```python
from build123d import *

# Parameters (mm, degrees)
F0_R     = 22.425
F1_DEPTH = 1.5
F2_R     = 10.5
F3_DEPTH = 0.25
F4_R     = 4
F5_DEPTH = 48.25
F7_D     = 4
F9_D     = 4
F11_D    = 3.5
F13_D    = 4


with BuildPart() as f1:
    # F0 (on Front) → F1 (new body)
    with BuildSketch(Plane.XZ):
        Circle(F0_R)
    extrude(amount=F1_DEPTH)

    # F2 (on face) → F3 (join)
    with BuildSketch(Plane.XZ.offset(1.5)):
        Circle(F2_R)
    extrude(amount=F3_DEPTH)

    # F4 (on face) → F5 (join)
    with BuildSketch(Plane.XZ.offset(1.75)):
        Circle(F4_R)
    extrude(amount=F5_DEPTH)

    # F7 (through all)
    with Locations(Plane(origin=(0, 0, 0), x_dir=(0, 1, 0), z_dir=(-1, 0, 0))):
        with Locations((-33, 0)):
            Hole(F7_D / 2)

    # F9 (through all)
    with Locations(Plane.YZ):
        with Locations((-33, 0)):
            Hole(F9_D / 2)

    # F11 (through all)
    with Locations(Plane(origin=(0, 0, 0), x_dir=(-1, 0, 0), z_dir=(0, 1, 0))):
        with Locations((0, 14.25), (-12.340862, -7.125), (12.340862, -7.125)):
            Hole(F11_D / 2)

    # F13 (through all)
    with Locations(Plane(origin=(0, 0, 0), x_dir=(-1, 0, 0), z_dir=(0, 1, 0))):
        with Locations((-15.155445, 8.75), (0, -17.5), (15.155445, 8.75)):
            Hole(F13_D / 2)


solid = f1.part
```
Design review of the part built by this model. Coordinates are the model's own, in mm. A direction names the side the tool comes from. Round coordinates to 2 decimals unless told otherwise and drop trailing zeros. Order: outer loops, then holes, each group sorted by start corner. A loop starts at its lowest first (then second) coordinate and runs counter-clockwise, first axis right, second up. Notation, with made-up numbers: M -35.5,56.5 L 3.5,56.5 A38 ccw 3.5,94.5 Z; hole C -24,69 d1. An arc over 180 degrees is marked long. Put each result on its own line as item: value.
Q1. Machinability: for faces 1 (the face through (5, -1.5, -10)), 2 (the face through (-15.416, -0.76, 10.733)), which of the approach directions +Z, -Z, +X, -X, +Y, -Y give a long, thin tool a straight path to every point of the face, cutting with its end or side? Answer none if there is none.
Reported:
face 1: -Y
face 2: +Y, -Y
Q2. Consider section B-B (x = -12). State the section outline as (y, z) points.
Reported:
outline: M -1.5,-18.94 L 0,-18.94 L 0,-8.84 L -1.5,-8.84 Z; M -1.5,-5.41 L 0,-5.41 L 0,18.94 L -1.5,18.94 Z
Q3. Consider section D-D (x = -7.5). State the section outline as (y, z) points, and give its area (3 significant figures).
Reported:
outline: M -1.75,-7.35 L -1.5,-7.35 L -1.5,-21.13 L 0,-21.13 L 0,21.13 L -1.5,21.13 L -1.5,7.35 L -1.75,7.35 Z
area: 67.1 mm²
Q4. Draft analysis for pull direction Z (two halves, no side actions). For faces 3 (the face through (17.063, -0.76, 9.351)), 4 (the face through (0, 0, 0)), 5 (the face through (-0.867, -25.537, -3.905)), state which applies: released by +Z, released by -Z, zero draft, split by the parting line, or undercut.
Reported:
face 3: undercut
face 4: zero draft
face 5: split by the parting line
Q5. To check wall thickness, follow line 1 (Z direction, x = 0, y = -0.6) (3 decimals); line 2 (Y direction, x = 3, z = -6); line 3 (Y direction, x = -7.5, z = -15.5). State the ranges of each line that lie inside material, in increasing order.
Reported:
line 1: -22.425 to -19.5, -15.5 to 12.5, 16 to 22.425
line 2: -1.75 to 0
line 3: -1.5 to 0
Q6. Insertion check: pin 1 Ø5 at (x, z) = (-15.16, 8.75) entering from +Y; pin 2 Ø4.5 at (x, z) = (15.16, 8.75) entering from -Y; pin 3 Ø6.5 at (y, z) = (-33, 0) entering from -X; pin 4 Ø8 at (x, y) = (2, -7.5) entering from -Z. Each pin has a flat end and moves straight along its axis. Give the tip position at first contact, or say it passes through.
Reported:
pin 1: y = 0
pin 2: y = -1.5
pin 3: x = -4
pin 4: z = -4
Q7. Consider section C-C (y = -33). State the section outline as (x, z) points.
Reported:
outline: M -3.46,-2 A4 ccw 3.46,-2 Z; M -3.46,2 L 3.46,2 A4 ccw Z
Q8. Consider section A-A (z = 0). State the section outline as (x, y) points (3 decimals), and give its area (3 significant figures).
Reported:
outline: M -22.425,-1.5 L -10.5,-1.5 L -10.5,-1.75 L -4,-1.75 L -4,-31 L 4,-31 L 4,-1.75 L 10.5,-1.75 L 10.5,-1.5 L 22.425,-1.5 L 22.425,0 L -22.425,0 Z; M -4,-50 L 4,-50 L 4,-35 L -4,-35 Z
area: 427 mm²
